CAD build for the part. Positions are in the model's coordinates, mm. Face numbers are marked on the shaded views. A direction names the side the tool comes from. Coordinates: 2 decimals unless noted, no trailing zeros. Loops run counter-clockwise (first coordinate to the right, second up) from the corner with the lowest first, then second, coordinate; pieces in that order, holes last. Notation, with made-up numbers: (25.5, -38.5) -> (58.5, -38.5) arc R18 cw to (58.5, -21.5) -> close; hole circle Ø5 at (-12.5, -14). An arc over 180 degrees is marked (long way). Answer as a JSON object with one key per item and string values. Group by question number.
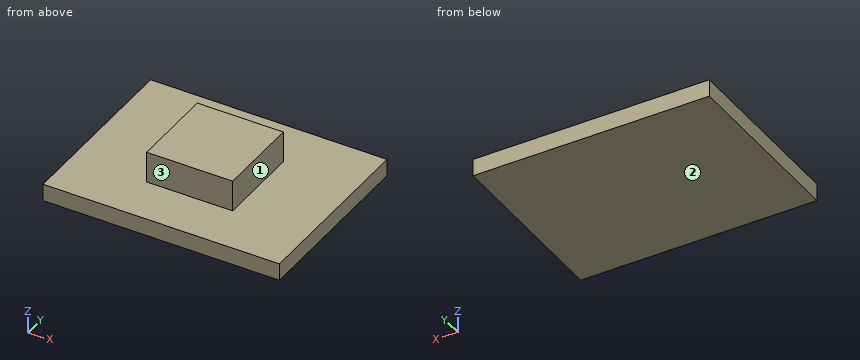
from build123d import *

# Parameters (mm, degrees)
SKETCH1_W      = 22
SKETCH1_H      = 17
PCB_DEPTH      = 1.6
SKETCH2_W      = 8
SKETCH2_H      = 8
INDUCTOR_DEPTH = 2.9


with BuildPart() as part:
    # Sketch1 → PCB (new body)
    with BuildSketch(Plane.XY):
        Rectangle(SKETCH1_W, SKETCH1_H)
    extrude(amount=PCB_DEPTH)

    # Sketch2 → Inductor (add)
    with BuildSketch(Plane.XY.offset(1.6)):
        Rectangle(SKETCH2_W, SKETCH2_H)
    extrude(amount=INDUCTOR_DEPTH)


solid = part.part
Item 1: Drill centre lines: L1, parallel to Y at x = -3.75, z = 3.7; L2, parallel to Z at x = -1.25, y = 8. Where is each one in solid material? Low to high.
Item 2: Band-saw the part on C-C, the plane z = 3. List the corners of the cut face in (x, y).
Item 3: Flat gauge pins, fed straight in: P1, Ø2, axis at x = -4, z = 3.5, coming from the -Y side; P2, Ø1.5, axis at y = -1.5, z = 2.5, coming from the +X side. Where does each tip first touch, or does it go through?
Item 4: Band-saw the part on A-A, the plane x = -1. List the corners of the cut face in (y, z).
Item 5: Band-saw the part on B-B, the plane y = 3.25. List the corners of the cut face in (x, z).
Item 6: 3-axis set-ups, long thin cutter, end or side, ignore diameter. For the marked faces 1, 2 and 3: which of +Z, -Z, +X, -X, +Y, -Y reach the whole face in a straight line?
Item 7: Band-saw the part on D-D, the plane x = 8.5. List the corners of the cut face in (y, z).
Reply:
{
 "1": {"L1": "-4 to 4", "L2": "0 to 1.6"},
 "2": {"outline": "(-4, -4) -> (4, -4) -> (4, 4) -> (-4, 4) -> close"},
 "3": {"P1": "y = -4", "P2": "x = 4"},
 "4": {"outline": "(-8.5, 0) -> (8.5, 0) -> (8.5, 1.6) -> (4, 1.6) -> (4, 4.5) -> (-4, 4.5) -> (-4, 1.6) -> (-8.5, 1.6) -> close"},
 "5": {"outline": "(-11, 0) -> (11, 0) -> (11, 1.6) -> (4, 1.6) -> (4, 4.5) -> (-4, 4.5) -> (-4, 1.6) -> (-11, 1.6) -> close"},
 "6": {"face 1": "+Z, +X, +Y, -Y", "face 2": "-Z, +X, -X, +Y, -Y", "face 3": "+Z, +X, -X, -Y"},
 "7": {"outline": "(-8.5, 0) -> (8.5, 0) -> (8.5, 1.6) -> (-8.5, 1.6) -> close"}
}
